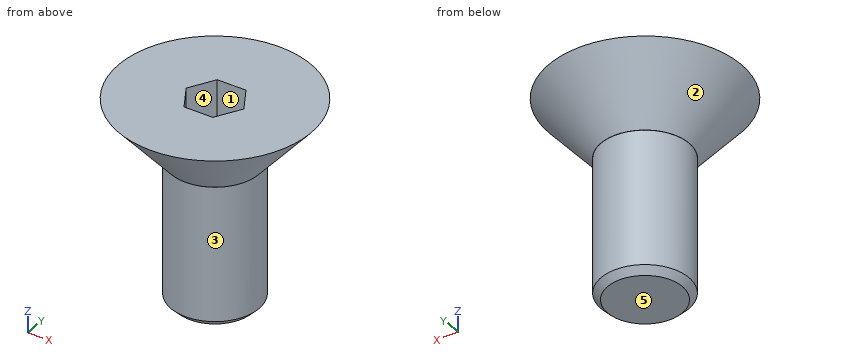
Solid Edge part; units mm, degrees
sketch "Sketch1" plane through (0, 0, 0) normal (0, 0, 1) x (1, 0, 0)
  circle A0 centre (0, 0) radius 4.5593
extrude "Protrusion1" add sketch "Sketch1" along normal blind 2.8448
sketch "Sketch2" plane through (0, 0, 0) normal (0, 0, -1) x (1, 0, 0)
  circle A0 centre (0, 0) radius 2.0828
extrude "Protrusion2" add sketch "Sketch2" along normal blind 6.6802
sketch "Sketch3" plane through (0, 0, -6.6802) normal (0, 0, -1) x (1, 0, 0)
  circle A0 centre (0, 0) radius 2.0825
extrude "Cutout1" cut sketch "Sketch3" against normal blind 6.6735 flip side to cut
chamfer "Chamfer_1" distance 0.3124 angle 45 1 edges at (-2.0825, 0, -6.6802)
sketch "Sketch4" plane through (0, 0, 2.8448) normal (0, 0, 1) x (1, 0, 0)
  line L0 (-0.6874, 1.1906) -> (0.6874, 1.1906)
  line L1 (1.3748, 0) -> (0.6874, 1.1906)
  line L2 (0.6874, -1.1906) -> (1.3748, 0)
  line L3 (-0.6874, -1.1906) -> (0.6874, -1.1906)
  line L4 (-1.3748, 0) -> (-0.6874, -1.1906)
  line L5 (-0.6874, 1.1906) -> (-1.3748, 0)
extrude "Cutout2" cut sketch "Sketch4" against normal blind 1.8965
sketch "Sketch5" plane through (0, 0, 0) normal (0, -1, 0) x (1, 0, 0)
  line L0 (4.5593, 2.8448) -> (2.0864, 0)
  line L1 (2.0864, 0) -> (4.5593, 0)
  line L2 (4.5593, 0) -> (4.5593, 2.8448)
revolve "RevolvedCutout1" cut sketch "Sketch5" angle 360 about axis through (0, 0, 14.0017) along (0, 0, -1)
properties part number "166340"
The model under review builds one solid part; all positions refer to its coordinate system, in mm. Face numbers are marked on the shaded views. A direction names the side the tool comes from. Give positions to 0.01 mm unless a question says otherwise; leave off trailing zeros. Order: outer loops, then holes, each group sorted by start corner. A loop starts at its lowest first (then second) coordinate and runs counter-clockwise, first axis right, second up. Notation, with made-up numbers: M 41,-8.5 L 68,-8.5 A16 cw 68,11.5 Z; hole C -16.75,-20 d11. An arc over 180 degrees is marked long. Use one line per item in the form item = value. Start each with the question number.
Item 1: Insertion check: pin 1 Ø1 at (x, z) = (-2, -4.5) entering from +Y; pin 2 Ø4 at (y, z) = (-0.5, -4) entering from -X; pin 3 Ø3 at (y, z) = (-3, -1) entering from -X. Each pin has a flat end and moves straight along its axis. Give the tip position at first contact, or say it passes through.
Item 2: The part is to be moulded in two halves that separate along Y. For the marked faces 3, 4 and 5, say which applies: pulls with the +Y half, pulls with the -Y half, needs draft (parallel to the pull), parting line crosses it, or undercut.
Item 3: We need section B-B on z = -3.75. Give the boundary of the cut face in (x, y) (1 decimal), plus the area to 3 significant figures.
Item 4: For the marked faces 1 and 2, list the 3-axis set-ups (+Z, -Z, +X, -X, +Y, -Y) from which the entire face can be reached by the end or side of a thin tool; tool diameter is ignored.
Item 5: To check wall thickness, follow line 1 along Y through (x, z) = (0, -4.5); line 2 along X through (y, z) = (3, 2.75); line 3 along Y through (x, z) = (0.5, -3). State the ranges of each line that lie inside material, in increasing order. Write a range as from..to.
Completed:
q1.pin_1 = 1.44
q1.pin_2 = -2.08
q1.pin_3 = -1.44
q2.face_3 = parting line crosses it
q2.face_4 = undercut
q2.face_5 = needs draft
q3.outline = C 0,0 d4.2
q3.area = 13.6 mm²
q4.face_1 = +Z
q4.face_2 = -Z
q5.line_1 = -2.08..2.08
q5.line_2 = -3.32..3.32
q5.line_3 = -2.02..2.02
